Read the model definition and answer for the solid it produces. Units are mm, in the model's axes. Face numbers are marked on the shaded views. Give positions to 0.01 mm unless a question says otherwise; leave off trailing zeros. Order: outer loops, then holes, each group sorted by start corner. A loop starts at its lowest first (then second) coordinate and runs counter-clockwise, first axis right, second up. Notation, with made-up numbers: M -19,6 L 10,6 A27 ccw 10,23 Z; hole C -10,76 d11. An arc over 180 degrees is marked long. One line per item, written item: value.
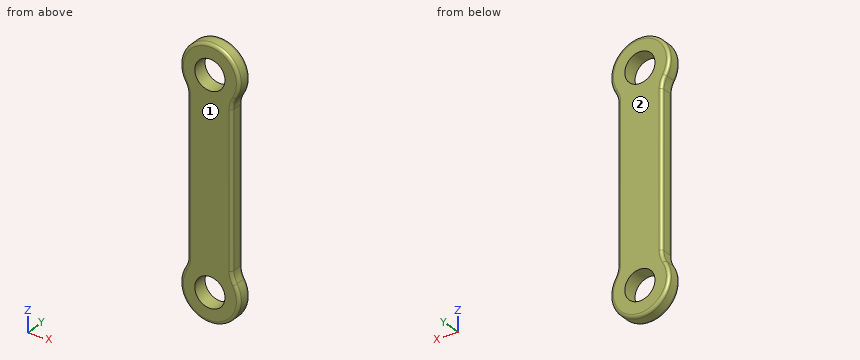
Autodesk Inventor part; units mm, degrees
ref_plane "YZ Plane" through (0, 0, 0) normal (1, 0, 0) x (0, 1, 0)
ref_plane "XZ Plane" through (0, 0, 0) normal (0, 1, 0) x (-1, 0, 0)
ref_plane "XY Plane" through (0, 0, 0) normal (0, 0, 1) x (1, 0, 0)
sketch "Sketch1" plane through (0, 0, 0) normal (0, 1, 0) x (-1, 0, 0)
  circle A0 centre (0, 0) radius 3.2512
  circle A1 centre (0, -44.45) radius 3.2512
  circle A2 centre (0, 0) radius 6.35 construction
  circle A3 centre (0, -44.45) radius 6.35 construction
  line L0 (0, -6.35) -> (0, -38.1) construction
  line L1 (4.7625, -5.7238) -> (4.7625, -38.7262)
  line L2 (-4.7625, -5.7238) -> (-4.7625, -38.7262)
  arc A4 (5.4429, -3.2708) -> (-5.4429, -3.2708) centre (0, 0) ccw
  arc A5 (-5.4429, -41.1792) -> (5.4429, -41.1792) centre (0, -44.45) ccw
  arc A6 (5.4429, -3.2708) -> (4.7625, -5.7238) centre (9.525, -5.7238) ccw
  arc A7 (-4.7625, -5.7238) -> (-5.4429, -3.2708) centre (-9.525, -5.7238) ccw
  arc A8 (-5.4429, -41.1792) -> (-4.7625, -38.7262) centre (-9.525, -38.7262) ccw
  arc A9 (4.7625, -38.7262) -> (5.4429, -41.1792) centre (9.525, -38.7262) ccw
  point P0 (4.7625, -4.2001)
  point P1 (4.7625, -40.2499)
  point P2 (-4.7625, -4.2001)
  point P3 (-4.7625, -40.2499)
  dimension "d0" = 6.5024
  dimension "d1" = 44.45
  dimension "d2" = 12.7
  dimension "d3" = 4.7625
  dimension "d4" = 4.7625
  dimension "d5" = 4.7625
extrude "Extrusion1" add sketch "Sketch1" along normal blind 3.175
fillet "Fillet1" radius 0.635 16 edges at (-4.9357, 3.175, -4.451) (0, 3.175, 6.35) (4.9357, 3.175, -4.451) (4.7625, 3.175, -22.225) (4.9357, 3.175, -39.999) (0, 3.175, -50.8) (-4.9357, 3.175, -39.999) (-4.7625, 3.175, -22.225) (-4.9357, 0, -4.451) (0, 0, 6.35) (4.9357, 0, -4.451) (4.7625, 0, -22.225) (4.9357, 0, -39.999) (0, 0, -50.8) (-4.9357, 0, -39.999) (-4.7625, 0, -22.225)
properties part number "ELEV_044_CFSPRINGHOLDER" material "Aluminum 6061"
1) Find section A-A, the plane z = -44.45. Write down the section's boundary in (x, y) (3 decimals), plus the area to 3 significant figures.
Reported:
outline: M -6.35,0.635 A0.635 ccw -5.715,0 L -3.251,0 L -3.251,3.175 L -5.715,3.175 A0.635 ccw -6.35,2.54 Z; M 3.251,0 L 5.715,0 A0.635 ccw 6.35,0.635 L 6.35,2.54 A0.635 ccw 5.715,3.175 L 3.251,3.175 Z
area: 19.3 mm^2
2) Each of these flat-tipped pins is pushed along its axis until it touches: pin 1 Ø1 at (x, y) = (-5, 1.5) entering from -Z; pin 2 Ø1.5 at (x, y) = (1, 1.5) entering from +Z; pin 3 Ø4 at (x, z) = (0, 0) entering from +Y; pin 4 Ø1 at (y, z) = (1, -26.5) entering from -X. Where does it stop, or does it pass through?
Reported:
pin 1: stops at z = -48.93
pin 2: stops at z = 6.35
pin 3: passes through
pin 4: stops at x = -4.76
3) Find section C-C, the plane y = 1.7. Write down the section's boundary in (x, z).
Reported:
outline: M -5.44,-41.18 A6.35 ccw long 5.44,-41.18 A4.76 cw 4.76,-38.73 L 4.76,-5.72 A4.76 cw 5.44,-3.27 A6.35 ccw long -5.44,-3.27 A4.76 cw -4.76,-5.72 L -4.76,-38.73 A4.76 cw Z; hole C 0,-44.45 d6.5; hole C 0,0 d6.5
4) Find section D-D, the plane z = -16.5. Write down the section's boundary in (x, y) (1 decimal).
Reported:
outline: M -4.8,0.6 A0.6 ccw -4.1,0 L 4.1,0 A0.6 ccw 4.8,0.6 L 4.8,2.5 A0.6 ccw 4.1,3.2 L -4.1,3.2 A0.6 ccw -4.8,2.5 Z
5) Consider probe 1 along Z at (x, y) = (0, 0.95); probe 2 along Z at (x, y) = (0.25, 1.6); probe 3 along X at (y, z) = (1.95, -23.5). Determine where each line is inside the solid, lowest interval first.
Reported:
probe 1: z = -50.8 to -47.7, -41.2 to -3.25, 3.25 to 6.35
probe 2: z = -50.8 to -47.69, -41.21 to -3.24, 3.24 to 6.35
probe 3: x = -4.76 to 4.76
6) Find section B-B, the plane x = 0. Write down the section's boundary in (y, z) (3 decimals), plus the area to 3 significant figures.
Reported:
outline: M 0,-50.165 A0.635 ccw 0.635,-50.8 L 2.54,-50.8 A0.635 ccw 3.175,-50.165 L 3.175,-47.701 L 0,-47.701 Z; M 0,-41.199 L 3.175,-41.199 L 3.175,-3.251 L 0,-3.251 Z; M 0,3.251 L 3.175,3.251 L 3.175,5.715 A0.635 ccw 2.54,6.35 L 0.635,6.35 A0.635 ccw 0,5.715 Z
area: 140 mm^2
7) Determine the mould class of the marked faces 1 and 2 for opening direction Y: +Y half, -Y half, draft (parallel to the pull), parting line (faces both ways), or undercut.
Reported:
face 1: -Y half
face 2: +Y half
